Solid Edge part; units mm, degrees
sketch "Sketch1" plane through (0, 0, 0) normal (0, 0, 1) x (1, 0, 0)
  line L0 (-105, -61.5) -> (105, -61.5)
  line L1 (105, -61.5) -> (105, 61.5)
  line L2 (105, 61.5) -> (-105, 61.5)
  line L3 (-105, 61.5) -> (-105, -61.5)
  dimension "D1" = 105
  dimension "D2" = 105
extrude "Protrusion1" add sketch "Sketch1" along normal blind 2
hole "Hole1" at (-1, -57.5, 2) direction (0, 0, -1) diameter 0.8 end through all
hole "Hole2" at (-26, -57.5, 2) direction (0, 0, -1) diameter 0.8 end through all
sketch "Sketch2" plane through (0, 0, 2) normal (0, 0, 1) x (-1, 0, 0)
  line L0 (-0.25, 61) -> (0.25, 61)
  line L1 (0.25, 61) -> (0.25, 61.5)
  line L2 (0.25, 61.5) -> (-0.25, 61.5)
  line L3 (-0.25, 61.5) -> (-0.25, 61)
  dimension "D1" = 0.25
extrude "Cutout1" cut sketch "Sketch2" against normal through all
sketch "Sketch3" plane through (0, 0, 2) normal (0, 0, 1) x (1, 0, 0)
  line L0 (105, -61.5) -> (105, 61.5)
  line L1 (49, -61.5) -> (105, -61.5)
  line L2 (49, 3.5) -> (49, -61.5)
  line L3 (58, 3.5) -> (49, 3.5)
  line L4 (58, 23.5) -> (58, 3.5)
  line L5 (49, 23.5) -> (58, 23.5)
  line L6 (49, 61.5) -> (49, 23.5)
  line L7 (105, 61.5) -> (49, 61.5)
  dimension "D1" = 58
  dimension "D2" = 49
  dimension "D3" = 49
extrude "Ausschnitt_3" cut sketch "Sketch3" against normal blind 2
hole "Hole3" at (-98.5, 55.5, 2) direction (0, 0, -1) diameter 3.5 end through all
hole "Hole4" at (44, 55.5, 2) direction (0, 0, -1) diameter 3.5 end through all
hole "Hole5" at (44, -48.5, 2) direction (0, 0, -1) diameter 3.5 end through all
hole "Hole6" at (-18, -56.5, 2) direction (0, 0, -1) diameter 3.5 end through all
hole "Hole7" at (-98.5, -56.5, 2) direction (0, 0, -1) diameter 3.5 end through all
hole "Hole8" at (44, -0.5, 2) direction (0, 0, -1) diameter 3.5 end through all
hole "Hole9" at (45, -42.5, 2) direction (0, 0, -1) diameter 1 end through all
hole "Hole10" at (45, 41.5, 2) direction (0, 0, -1) diameter 1 end through all
hole "Hole11" at (51, 13.5, 2) direction (0, 0, -1) diameter 1 end through all
hole "Hole12" at (-59.5, -36.5, 2) direction (0, 0, -1) diameter 1 end through all
hole "Hole13" at (-49, -36.5, 2) direction (0, 0, -1) diameter 1 end through all
hole "Hole14" at (-70, -36.5, 2) direction (0, 0, -1) diameter 1 end through all
hole "Hole15" at (31, 28.5, 2) direction (0, 0, -1) diameter 4.3 end up to next
hole "Hole16" at (31, -41.5, 2) direction (0, 0, -1) diameter 4.3 end up to next
hole "Hole17" at (-14, -41.5, 2) direction (0, 0, -1) diameter 4.3 end up to next
hole "Hole18" at (-14, 28.5, 2) direction (0, 0, -1) diameter 4.3 end up to next
hole "Hole19" at (8.5, -41.5, 2) direction (0, 0, -1) diameter 0.2 end through all
hole "Hole20" at (8.5, 28.5, 2) direction (0, 0, -1) diameter 0.2 end through all
sketch "Sketch4" plane through (-23.4888, 0, 2) normal (0, 0, 1) x (1, 0, 0)
  line L0 (9.7388, -61.5) -> (10.2388, -61.5)
  line L1 (10.2388, -61.5) -> (10.2388, -61)
  line L2 (10.2388, -61) -> (9.7388, -61)
  line L3 (9.7388, -61) -> (9.7388, -61.5)
  dimension "D1" = 10.2388
extrude "Cutout2" cut sketch "Sketch4" against normal through all
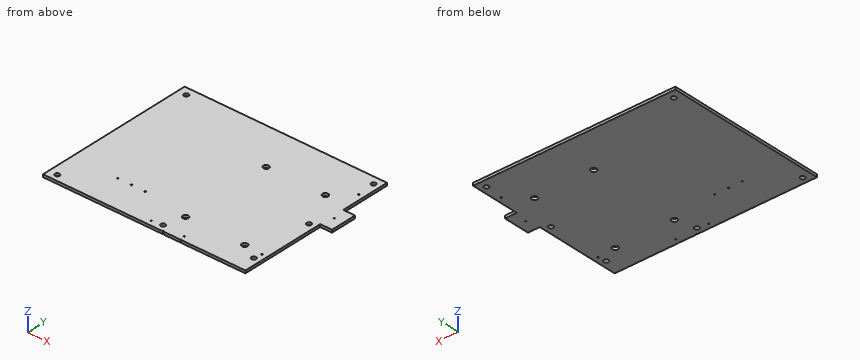
Could you check a few things on this model? Use its own coordinates, in mm. Coordinates: 2 decimals unless noted, no trailing zeros. Write each loop counter-clockwise with the first axis right and the second up, starting at its lowest first coordinate (ties: lowest second). Pieces come first, ordered by that corner, then holes. Notation, with made-up numbers: (16.25, 80) -> (43.25, 80) arc R29 cw to (43.25, 110) -> close; hole circle Ø2 at (50, -14.5). An arc over 180 degrees is marked (long way). Write item = value, one per line. Start each with the question number.
(1) I want a section at A-A (x = -98.5). Please give me the cut outline in (y, z), plus the area to 3 significant figures.
(2) I need wall thicknesses on line 1 (Y direction, x = -14, z = 1.45); line 2 (X direction, y = -41.5, z = 0.85); line 3 (Y direction, x = 44, z = 1.5). Which ranges of each line are inside material? Lowest first, please. Write a range as [from, to].
(3) I want a section at B-B (y = -0.5). Please give me the cut outline in (x, z), plus the area to 3 significant figures.
(4) Will these pins go through, and if not, where does the flat tip stop? pin 1 (3.5 mm diameter, centred on x = -14, y = 28.5, fed in from -Z); pin 2 (1 mm diameter, centred on x = 52.5, z = 0.5, fed in from +Y); pin 3 (0.6 mm diameter, centred on y = 47.5, z = 1.5, fed in from +X).
(5) I want a section at C-C (x = -18). Please give me the cut outline in (y, z).
(6) I want a section at D-D (z = 1.55). Give the number of separate pieces and of enclosed holes in the cut face, plus the area to 3 significant figures.
Result set:
q1.outline = (-61.5, 0) -> (-58.25, 0) -> (-58.25, 2) -> (-61.5, 2) -> close; (-54.75, 0) -> (53.75, 0) -> (53.75, 2) -> (-54.75, 2) -> close; (57.25, 0) -> (61.5, 0) -> (61.5, 2) -> (57.25, 2) -> close
q1.area = 232 mm2
q2.line_1 = [-61.5, -43.65], [-39.35, 26.35], [30.65, 61.5]
q2.line_2 = [-105, -16.15], [-11.85, 8.4], [8.6, 28.85], [33.15, 49]
q2.line_3 = [-61.5, -50.25], [-46.75, -2.25], [1.25, 53.75], [57.25, 61.5]
q3.outline = (-105, 0) -> (42.25, 0) -> (42.25, 2) -> (-105, 2) -> close; (45.75, 0) -> (49, 0) -> (49, 2) -> (45.75, 2) -> close
q3.area = 301 mm2
q4.pin_1 = through
q4.pin_2 = 23.5
q4.pin_3 = 49
q5.outline = (-61.5, 0) -> (-58.25, 0) -> (-58.25, 2) -> (-61.5, 2) -> close; (-54.75, 0) -> (61.5, 0) -> (61.5, 2) -> (-54.75, 2) -> close
q6.separate_pieces = 1
q6.enclosed_holes = 20
q6.area = 19,000 mm2
